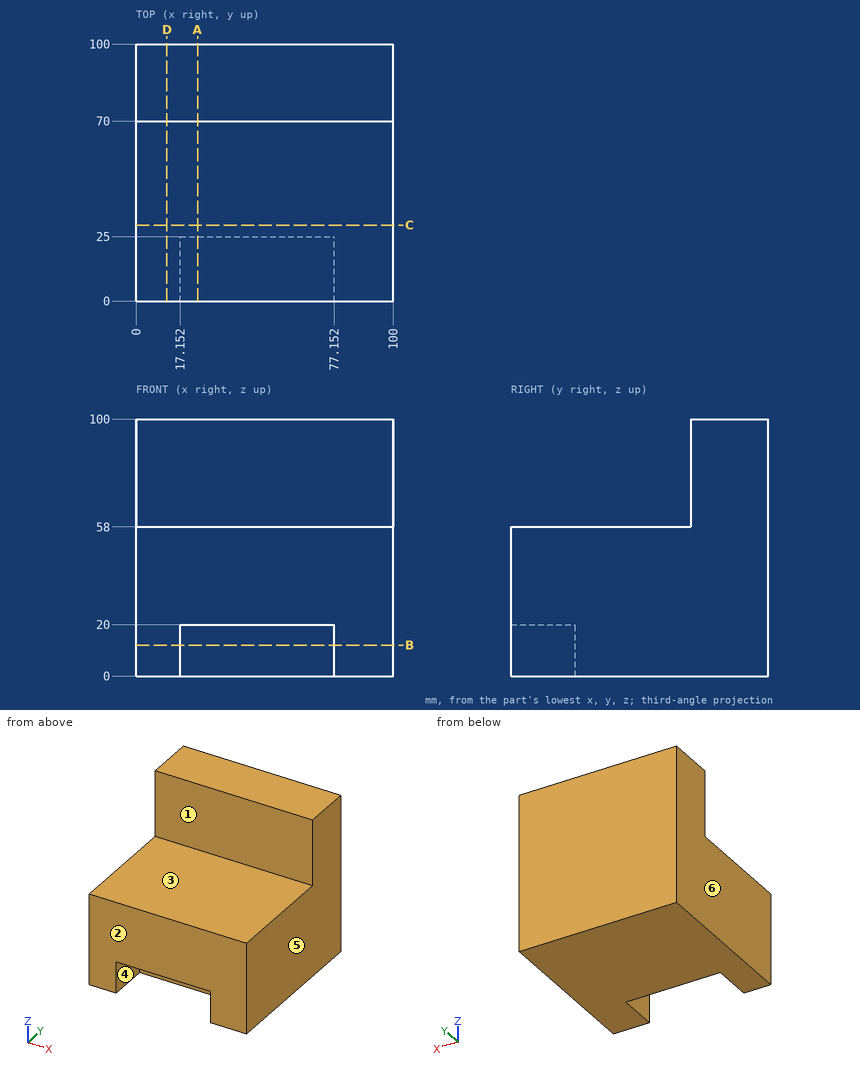
The figure shows three views and two pictorial views of one solid part (mm, origin at its lowest corner). Answer the questions. A direction names the side the tool comes from. Round coordinates to 2 decimals unless told otherwise and drop trailing zeros. Write each loop counter-clockwise with the first axis right and the second up, starting at its lowest first coordinate (ties: lowest second). Pieces come first, ordered by that corner, then holes. Notation, with made-up numbers: (23, 56.5) - (76, 56.5) arc R11 cw to (76, 67.5) - close; hole circle Ø5 at (10, 40). An arc over 180 degrees is marked (long way). Answer in a Markdown table with one row per item. Add a question column.
1. The mould has two halves that part along X. Classify the marked faces 3, 4, 5 and 6: +X half, -X half, draft (parallel to the pull), parting line (faces both ways), or undercut.
2. A cutting plane is placed at D-D, the plane x = 12. Determine the outline of the cut face in (y, z), and give its area (3 significant figures).
3. Find the intervals of material crossed by line 1 along Z through (x, y) = (47, 20.5); line 2 along Y through (x, z) = (65, 82); line 3 along Z through (x, y) = (17, 12), in increasing order. Write a range as from..to.
4. A cutting plane is placed at A-A, the plane x = 24. Determine the outline of the cut face in (y, z).
5. Given pin 1 (5 mm diameter, centred on x = 83.5, y = 24, fed in from +Z); pin 2 (21 mm diameter, centred on x = 72, z = 73, fed in from -Y), each flat-ended and moving along its own axis, determine where each tip first touches the part or whether it passes through.
6. For the marked faces 1 and 2, determine the directions among +Z, -Z, +X, -X, +Y, -Y from which every point of the face is accessible in a straight line to the end or side of a thin tool.
7. A cutting plane is placed at C-C, the plane y = 29.5. Determine the outline of the cut face in (x, z).
8. A cutting plane is placed at B-B, the plane z = 12. Determine the outline of the cut face in (x, y).
Worked out:
| question | item | result |
|---|---|---|
| 1 | face 3 | draft |
| 1 | face 4 | undercut |
| 1 | face 5 | +X half |
| 1 | face 6 | -X half |
| 2 | outline | (0, 0) - (100, 0) - (100, 100) - (70, 100) - (70, 58) - (0, 58) - close |
| 2 | area | 7,060 mm^2 |
| 3 | line 1 | 20..58 |
| 3 | line 2 | 70..100 |
| 3 | line 3 | 0..58 |
| 4 | outline | (0, 20) - (25, 20) - (25, 0) - (100, 0) - (100, 100) - (70, 100) - (70, 58) - (0, 58) - close |
| 5 | pin 1 | z = 58 |
| 5 | pin 2 | y = 70 |
| 6 | face 1 | +Z, +X, -X, -Y |
| 6 | face 2 | +Z, -Z, +X, -X, -Y |
| 7 | outline | (0, 0) - (100, 0) - (100, 58) - (0, 58) - close |
| 8 | outline | (0, 0) - (17.15, 0) - (17.15, 25) - (77.15, 25) - (77.15, 0) - (100, 0) - (100, 100) - (0, 100) - close |
